Could you check a few things on this model? Use its own coordinates, in mm. Round coordinates to 2 decimals unless told otherwise and drop trailing zeros. Loops run counter-clockwise (first coordinate to the right, second up) from the corner with the lowest first, then second, coordinate; pieces in that order, holes last. Notation, with made-up numbers: M -39.75,-2 L -3.75,-2 A25 cw -3.75,16 Z; hole C -8,64 d3. An arc over 180 degrees is marked long. One line per item, written item: value. Start each with the question number.
Q1. Imagine slicing it at B-B (z = 4.5). Please give me the cut outline in (x, y), then the cut area to 3 significant figures.
Q2. Imagine slicing it at A-A (x = 144.5). Please give me the cut outline in (y, z) (1 decimal), then the cut area to 3 significant figures.
Q3. Thinking about a two-plate mould opening in Z: for faces 1 (the face through (333, 104, -3.175)), 2 (the face through (333, 104, 0)), 3 (the face through (676.402, 100, -1)), which applies, released by +Z, released by -Z, zero draft, split by the parting line, or undercut?
Q4. Imagine slicing it at C-C (y = 140). Please give me the cut outline in (x, z) (3 decimals).
Q5. Please list where these lines run through material, in increasing order: line 1 along Y through (x, z) = (415, 2.25); line 2 along Z through (x, y) = (122, 28) (3 decimals); line 3 along Y through (x, z) = (319.5, -1.5).
Q6. I'm going to push flat-ended pins straight in: pin 1 Ø2 at (x, z) = (113, 0) entering from -Y; pin 2 Ø10 at (x, y) = (476.5, 175) entering from +Z. Where does each tip first touch, or does it pass through?
from build123d import *

# Parameters (mm, degrees)
SKETCH1_W          = 676.402
SKETCH1_H          = 204.15504
BASE_FLANGE1_DEPTH = 3.175
EDGE_FLANGE1_DEPTH = 676.402
SKETCH9_R          = 9.525
CUT_EXTRUDE1_DEPTH = 3.175


# Sheet-metal steps are written as plain solids
with BuildPart() as part:
    # Sketch1 → Base-Flange1 (new body)
    with BuildSketch(Plane.XY):
        with Locations((338.201, 102.07752)):
            Rectangle(SKETCH1_W, SKETCH1_H)
    extrude(amount=-BASE_FLANGE1_DEPTH)

    # Edge-Flange1 section (across the edge) → Edge-Flange1 (add)
    with BuildSketch(Plane(origin=(0, -1.5875, 0), x_dir=(0, 1, 0), z_dir=(1, 0, 0))):
        with BuildLine():
            Line((-3.175, 1.5875), (-3.175, 9.525))
            Line((-3.175, 9.525), (0, 9.525))
            Line((0, 9.525), (0, 1.5875))
            ThreePointArc((0, 1.5875), (0.464967985, 0.464967985), (1.5875, 0))
            Line((1.5875, 0), (1.5875, -3.175))
            ThreePointArc((1.5875, -3.175), (-1.780096045, -1.780096045), (-3.175, 1.5875))
        make_face()
    extrude(amount=EDGE_FLANGE1_DEPTH)

    # Sketch9 → Cut-Extrude1 (cut)
    with BuildSketch(Plane(origin=(0, 0, 1.251039998), x_dir=(-1, 0, 0), z_dir=(0, 0, -1))):
        with Locations((-267.508853456, 43.732259818)):
            Circle(SKETCH9_R)
        with Locations((-180.176306543, 43.732259818)):
            Circle(SKETCH9_R)
        with Locations((-38.908853456, 43.732259818)):
            Circle(SKETCH9_R)
        with Locations((-637.376306543, 43.732259818)):
            Circle(SKETCH9_R)
        with Locations((-496.108853456, 43.732259818)):
            Circle(SKETCH9_R)
        with Locations((-408.776306543, 43.732259818)):
            Circle(SKETCH9_R)
        with Locations((-38.908853456, 163.597780182)):
            Circle(SKETCH9_R)
        with Locations((-180.176306543, 163.597780182)):
            Circle(SKETCH9_R)
        with Locations((-408.776306543, 163.597780182)):
            Circle(SKETCH9_R)
        with Locations((-267.508853456, 163.597780182)):
            Circle(SKETCH9_R)
        with Locations((-637.376306543, 163.597780182)):
            Circle(SKETCH9_R)
        with Locations((-496.108853456, 163.597780182)):
            Circle(SKETCH9_R)
    extrude(amount=-CUT_EXTRUDE1_DEPTH, mode=Mode.SUBTRACT)


solid = part.part
Report:
1. outline: M 0,-4.76 L 676.4,-4.76 L 676.4,-1.59 L 0,-1.59 Z
1. area: 2,150 mm²
2. outline: M -4.8,1.6 A4.8 ccw 0,-3.2 L 204.2,-3.2 L 204.2,0 L 0,0 A1.6 cw -1.6,1.6 L -1.6,9.5 L -4.8,9.5 Z
2. area: 689 mm²
3. face 1: released by -Z
3. face 2: released by +Z
3. face 3: zero draft
4. outline: M 0,-3.175 L 676.402,-3.175 L 676.402,0 L 0,0 Z
5. line 1: y = -4.76 to -1.59
5. line 2: z = -3.175 to 0
5. line 3: y = -3.63 to 204.16
6. pin 1: stops at y = -4.73
6. pin 2: stops at z = 0
